from build123d import *

# Parameters (mm, degrees)
SKETCH3_W                      = 68
SKETCH3_H                      = 64
BASE_FLANGE1_DEPTH             = 3
EDGE_FLANGE1_STRIP_W           = 13.4732
EDGE_FLANGE1_STRIP_H           = 3
EDGE_FLANGE1_STRIP_CUT_DEPTH   = 9
EDGE_FLANGE1_STRIP_2_W         = 13.4732
EDGE_FLANGE1_STRIP_2_H         = 3
EDGE_FLANGE1_STRIP_CUT_2_DEPTH = 9
EDGE_FLANGE1_STRIP_3_W         = 13.4732
EDGE_FLANGE1_STRIP_3_H         = 3
EDGE_FLANGE1_STRIP_CUT_3_DEPTH = 9
EDGE_FLANGE1_STRIP_4_W         = 13.4732
EDGE_FLANGE1_STRIP_4_H         = 3
EDGE_FLANGE1_STRIP_CUT_4_DEPTH = 9
EDGE_FLANGE1_DEPTH             = 9
EDGE_FLANGE1_BEND_DEPTH        = 9
EDGE_FLANGE1_BEND_2_DEPTH      = 9
EDGE_FLANGE1_BEND_3_DEPTH      = 9
FILLET1_R                      = 3
FILLET2_R                      = 3
SKETCH20_R                     = 1.55
CUT_EXTRUDE1_DEPTH             = 109.701425934
SKETCH22_R                     = 1.35
CUT_EXTRUDE2_DEPTH             = 71.0285656


# Sheet-metal steps are written as plain solids
with BuildPart() as part:
    # Sketch3 → Base-Flange1 (new body)
    with BuildSketch(Plane(origin=(0, 0, 0), x_dir=(1, 0, 0), z_dir=(0, 1, 0))):
        Polygon((50, 31), (44, 31), (44, 48), (35, 48), (35, 42), (-35, 42), (-35, 48), (-44, 48), (-44, 31), (-50, 31), (-50, -31), (-44, -31), (-44, -48), (-35, -48), (-35, -42), (35, -42), (35, -48), (44, -48), (44, -31), (50, -31), align=None)
        Rectangle(SKETCH3_W, SKETCH3_H, mode=Mode.SUBTRACT)
    extrude(amount=-BASE_FLANGE1_DEPTH)

    # Edge-Flange1 strip (across the edge) → Edge-Flange1 strip cut (cut)
    with BuildSketch(Plane(origin=(-35, -3, 48), x_dir=(0, 0, -1), z_dir=(-1, 0, 0))):
        with Locations((-3, -1.5)):
            Rectangle(EDGE_FLANGE1_STRIP_W, EDGE_FLANGE1_STRIP_H)
    extrude(amount=EDGE_FLANGE1_STRIP_CUT_DEPTH, mode=Mode.SUBTRACT)

    # Edge-Flange1 strip 2 (across the edge) → Edge-Flange1 strip cut 2 (cut)
    with BuildSketch(Plane(origin=(44, -3, 48), x_dir=(0, 0, -1), z_dir=(-1, 0, 0))):
        with Locations((-3, -1.5)):
            Rectangle(EDGE_FLANGE1_STRIP_2_W, EDGE_FLANGE1_STRIP_2_H)
    extrude(amount=EDGE_FLANGE1_STRIP_CUT_2_DEPTH, mode=Mode.SUBTRACT)

    # Edge-Flange1 strip 3 (across the edge) → Edge-Flange1 strip cut 3 (cut)
    with BuildSketch(Plane(origin=(35, -3, -48), x_dir=(0, 0, 1), z_dir=(1, 0, 0))):
        with Locations((-3, -1.5)):
            Rectangle(EDGE_FLANGE1_STRIP_3_W, EDGE_FLANGE1_STRIP_3_H)
    extrude(amount=EDGE_FLANGE1_STRIP_CUT_3_DEPTH, mode=Mode.SUBTRACT)

    # Edge-Flange1 strip 4 (across the edge) → Edge-Flange1 strip cut 4 (cut)
    with BuildSketch(Plane(origin=(-44, -3, -48), x_dir=(0, 0, 1), z_dir=(1, 0, 0))):
        with Locations((-3, -1.5)):
            Rectangle(EDGE_FLANGE1_STRIP_4_W, EDGE_FLANGE1_STRIP_4_H)
    extrude(amount=EDGE_FLANGE1_STRIP_CUT_4_DEPTH, mode=Mode.SUBTRACT)

    # Edge-Flange1 section (across the edge) → Edge-Flange1 (add)
    with BuildSketch(Plane(origin=(-35, -3, 48), x_dir=(0, 0, -1), z_dir=(-1, 0, 0))):
        with BuildLine():
            Line((0, 0.7366), (0, 7))
            Line((0, 7), (3, 7))
            Line((3, 7), (3, 0.7366))
            ThreePointArc((3, 0.7366), (3.215745145, 0.215745145), (3.7366, 0))
            Line((3.7366, 0), (3.7366, -3))
            ThreePointArc((3.7366, -3), (1.094424801, -1.905575199), (0, 0.7366))
        make_face()
    extrude(amount=EDGE_FLANGE1_DEPTH)

    # Edge-Flange1 section 2 (across the edge) → Edge-Flange1 bend (add)
    with BuildSketch(Plane(origin=(44, -3, 48), x_dir=(0, 0, -1), z_dir=(-1, 0, 0))):
        with BuildLine():
            Line((0, 0.7366), (0, 7))
            Line((0, 7), (3, 7))
            Line((3, 7), (3, 0.7366))
            ThreePointArc((3, 0.7366), (3.215745145, 0.215745145), (3.7366, 0))
            Line((3.7366, 0), (3.7366, -3))
            ThreePointArc((3.7366, -3), (1.094424801, -1.905575199), (0, 0.7366))
        make_face()
    extrude(amount=EDGE_FLANGE1_BEND_DEPTH)

    # Edge-Flange1 section 3 (across the edge) → Edge-Flange1 bend 2 (add)
    with BuildSketch(Plane(origin=(35, -3, -48), x_dir=(0, 0, 1), z_dir=(1, 0, 0))):
        with BuildLine():
            Line((0, 0.7366), (0, 7))
            Line((0, 7), (3, 7))
            Line((3, 7), (3, 0.7366))
            ThreePointArc((3, 0.7366), (3.215745145, 0.215745145), (3.7366, 0))
            Line((3.7366, 0), (3.7366, -3))
            ThreePointArc((3.7366, -3), (1.094424801, -1.905575199), (0, 0.7366))
        make_face()
    extrude(amount=EDGE_FLANGE1_BEND_2_DEPTH)

    # Edge-Flange1 section 4 (across the edge) → Edge-Flange1 bend 3 (add)
    with BuildSketch(Plane(origin=(-44, -3, -48), x_dir=(0, 0, 1), z_dir=(1, 0, 0))):
        with BuildLine():
            Line((0, 0.7366), (0, 7))
            Line((0, 7), (3, 7))
            Line((3, 7), (3, 0.7366))
            ThreePointArc((3, 0.7366), (3.215745145, 0.215745145), (3.7366, 0))
            Line((3.7366, 0), (3.7366, -3))
            ThreePointArc((3.7366, -3), (1.094424801, -1.905575199), (0, 0.7366))
        make_face()
    extrude(amount=EDGE_FLANGE1_BEND_3_DEPTH)

    # Fillet1
    fillet1_edges = [part.edges().sort_by_distance(p)[0] for p in [
        (44, -1.5, 31),
        (-44, -1.5, 31),
        (-44, -1.5, -31),
        (44, -1.5, -31),
        (-34, -1.5, 32),
        (-34, -1.5, -32),
        (34, -1.5, -32),
        (34, -1.5, 32),
    ]]
    fillet(fillet1_edges, radius=FILLET1_R)

    # Fillet2
    fillet2_edges = [part.edges().sort_by_distance(p)[0] for p in [
        (50, -1.5, -31),
        (50, -1.5, 31),
        (-50, -1.5, 31),
        (-50, -1.5, -31),
    ]]
    fillet(fillet2_edges, radius=FILLET2_R - 0.0001)  # a hair under: the kernel refuses the full size

    # Sketch20 → Cut-Extrude1 (cut, through all)
    with BuildSketch(Plane.XY.offset(48)):
        with Locations((-39.5, -6.8683)):
            Circle(SKETCH20_R)
        with Locations((39.5, -6.8683)):
            Circle(SKETCH20_R)
    extrude(amount=-CUT_EXTRUDE1_DEPTH, mode=Mode.SUBTRACT)

    # Sketch22 → Cut-Extrude2 (cut, through all)
    with BuildSketch(Plane(origin=(0, 0, 0), x_dir=(1, 0, 0), z_dir=(0, 1, 0))):
        with Locations(Location((-45.8, 24.7, 0), (0, 0, 270))):
            Circle(SKETCH22_R)
        with Locations(Location((-45.8, -24.7, 0), (0, 0, 270))):
            Circle(SKETCH22_R)
        with Locations(Location((45.8, 24.7, 0), (0, 0, 270))):
            Circle(SKETCH22_R)
        with Locations(Location((45.8, -24.7, 0), (0, 0, 270))):
            Circle(SKETCH22_R)
    extrude(amount=-CUT_EXTRUDE2_DEPTH, mode=Mode.SUBTRACT)


solid = part.part
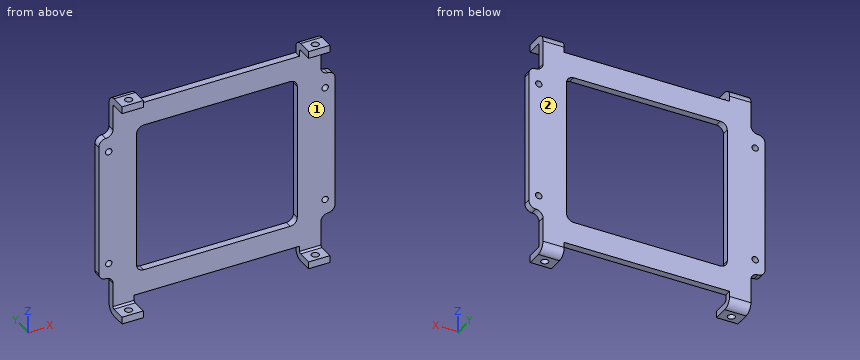
Could you check a few things on this model? Use its own coordinates, in mm. Face numbers are marked on the shaded views. Coordinates: 2 decimals unless noted, no trailing zeros. Order: outer loops, then holes, each group sorted by start corner. A loop starts at its lowest first (then second) coordinate and runs counter-clockwise, first axis right, second up. Notation, with made-up numbers: (56, -9.5) -> (89, -9.5) arc R9 ccw to (89, 4.5) -> close; hole circle Ø9 at (-24, 84). An arc over 180 degrees is marked (long way). One line per item, written item: value. Start each with the question number.
1) If I drill on L1, parallel to X at y = -2.35, z = -24.7; L2, parallel to Z at x = 28, y = -1.75; L3, parallel to X at y = -2.5, z = 7.5, over which ranges is the centre line in solid material (lowest first)? Write a range as [from, to].
2) Imagine slicing it at B-B on x = 39.5. List the corners of the cut face in (y, z) for me.
3) I'm going to push flat-ended pins straight in: pin 1 (5 mm diameter, centred on y = -7, z = -43.5, fed in from +X); pin 2 (3.5 mm diameter, centred on x = 45.8, z = -24.7, fed in from -Y); pin 3 (6 mm diameter, centred on x = 23, y = -3, fed in from +Z). Where does each tip first touch, or does it pass through?
4) Imagine slicing it at A-A on z = -24.7. List the corners of the cut face in (x, y) for me, plus the area to 3 significant figures.
5) We'd pull the mould along Z, two halves only. Please class the marked faces 1 and 2: +Z half, -Z half, draft (parallel to the pull), parting line (faces both ways), or undercut.
6) Imagine slicing it at C-C on x = 6. List the corners of the cut face in (y, z) for me, plus the area to 3 significant figures.
7) Imagine slicing it at D-D on y = -1.5. Count the separate pieces of the cut face and the enclosed holes in it, plus the area to 3 significant figures.
Answer list:
1. L1: x = [-50, -47.15], [-44.45, -34], [34, 44.45], [47.15, 50]
1. L2: z = [-42, -32], [32, 42]
1. L3: x = [-50, -34], [34, 50]
2. outline: (-10, -48) -> (-8.42, -48) -> (-8.42, -45) -> (-10, -45) -> close; (-10, 45) -> (-8.42, 45) -> (-8.42, 48) -> (-10, 48) -> close; (-5.32, -48) -> (-3.74, -48) arc R3.74 ccw to (0, -44.26) -> (0, 44.26) arc R3.74 ccw to (-3.74, 48) -> (-5.32, 48) -> (-5.32, 45) -> (-3.74, 45) arc R0.74 cw to (-3, 44.26) -> (-3, -44.26) arc R0.74 cw to (-3.74, -45) -> (-5.32, -45) -> close
3. pin 1: stops at x = 44
3. pin 2: stops at y = -3
3. pin 3: stops at z = 42
4. outline: (-50, -3) -> (-47.15, -3) -> (-47.15, 0) -> (-50, 0) -> close; (-44.45, -3) -> (-34, -3) -> (-34, 0) -> (-44.45, 0) -> close; (34, -3) -> (44.45, -3) -> (44.45, 0) -> (34, 0) -> close; (47.15, -3) -> (50, -3) -> (50, 0) -> (47.15, 0) -> close
4. area: 79.8 mm2
5. face 1: undercut
5. face 2: draft
6. outline: (-3, -42) -> (0, -42) -> (0, -32) -> (-3, -32) -> close; (-3, 32) -> (0, 32) -> (0, 42) -> (-3, 42) -> close
6. area: 60.0 mm2
7. separate pieces: 1
7. enclosed holes: 5
7. area: 3,960 mm2
